from build123d import *

# Parameters (mm, degrees)
SKETCH1_R           = 2.213186583
SKETCH1_R_2         = 2.28890728
BOSS_EXTRUDE1_DEPTH = 313


with BuildPart() as part:
    # Sketch1 → Boss-Extrude1 (new body)
    with BuildSketch(Plane(origin=(0, 0, 0), x_dir=(1, 0, 0), z_dir=(0, 1, 0))):
        Polygon((20, 0), (20, -7), (18, -7), (18, -4), (17, -4), (14, -7), (14, -13), (17, -16), (18, -16), (18, -13), (20, -13), (20, -27), (18, -27), (18, -24), (17, -24), (14, -27), (14, -33), (17, -36), (18, -36), (18, -33), (20, -33), (20, -40), (13, -40), (13, -38), (16, -38), (16, -37), (13, -34), (7, -34), (4, -37), (4, -38), (7, -38), (7, -40), (0, -40), (0, -33), (2, -33), (2, -36), (3, -36), (6, -33), (6, -27), (3, -24), (2, -24), (2, -27), (0, -27), (0, -13), (2, -13), (2, -16), (3, -16), (6, -13), (6, -7), (3, -4), (2, -4), (2, -7), (0, -7), (0, 0), (7, 0), (7, -2), (4, -2), (4, -3), (7, -6), (13, -6), (16, -3), (16, -2), (13, -2), (13, 0), align=None)
        with Locations(Location((10, -10, 0), (0, 0, 270))):
            Circle(SKETCH1_R, mode=Mode.SUBTRACT)
        with Locations(Location((10, -30, 0), (0, 0, 270))):
            Circle(SKETCH1_R_2, mode=Mode.SUBTRACT)
        Polygon((7, -14), (13, -14), (17, -18), (18, -18), (18, -22), (17, -22), (13, -26), (7, -26), (3, -22), (2, -22), (2, -18), (3, -18), align=None, mode=Mode.SUBTRACT)
    extrude(amount=BOSS_EXTRUDE1_DEPTH)


solid = part.part
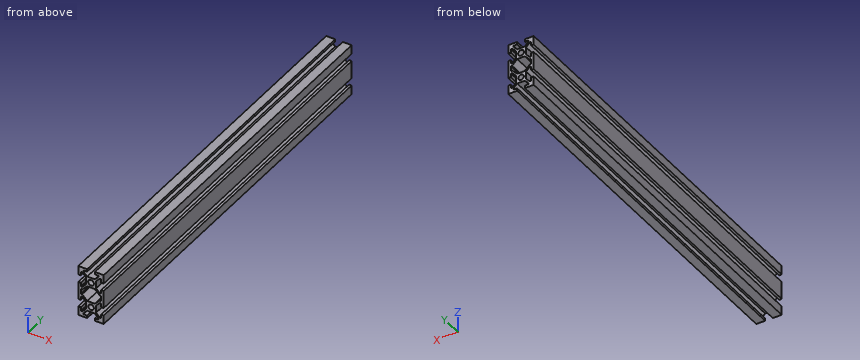
Geometry check sheet. Reference: the model listing, model coordinates, mm. Give positions to 0.01 mm unless a question says otherwise; leave off trailing zeros. Answer in a Markdown table with one row per item. Add a question column.
1) Cross-section at A-A on y = 71. State how many separate pieces and enclosed holes the cut face has, and give its area (3 significant figures).
2) Material ranges on probe 1 along Z at (x, y) = (17.25, 77.5); probe 2 along Z at (x, y) = (5, 56); probe 3 along Z at (x, y) = (1, 85.5), recorded low to high. Write a range as from..to.
3) Gauge pin test, flat ends, axial feed: P1, Ø3, axis at y = 149, z = 29.5, coming from the +X side; P2, Ø1.8, axis at x = 11, y = 80.5, coming from the +Z side; P3, Ø2, axis at x = 2.5, z = 28, coming from the -Y side; P4, Ø3, axis at x = 11, y = 178, coming from the -Z side. Record the tip position at first contact, or that the pin passes through.
Outcome:
| question | item | result |
|---|---|---|
| 1 | separate pieces | 1 |
| 1 | enclosed holes | 3 |
| 1 | area | 318 mm^2 |
| 2 | probe 1 | z = 0..4, 16..18, 22..24, 36..40 |
| 2 | probe 2 | z = 0..2, 4..6, 14..16, 24..26, 34..36, 38..40 |
| 2 | probe 3 | z = 0..7, 13..27, 33..40 |
| 3 | P1 | stops at x = 14 |
| 3 | P2 | stops at z = 34 |
| 3 | P3 | passes through |
| 3 | P4 | stops at z = 6 |
